The model under review builds one solid part; all positions refer to its coordinate system, in mm. Face numbers are marked on the shaded views. Round coordinates to 2 decimals unless told otherwise and drop trailing zeros. Order: outer loops, then holes, each group sorted by start corner. A loop starts at its lowest first (then second) coordinate and runs counter-clockwise, first axis right, second up.
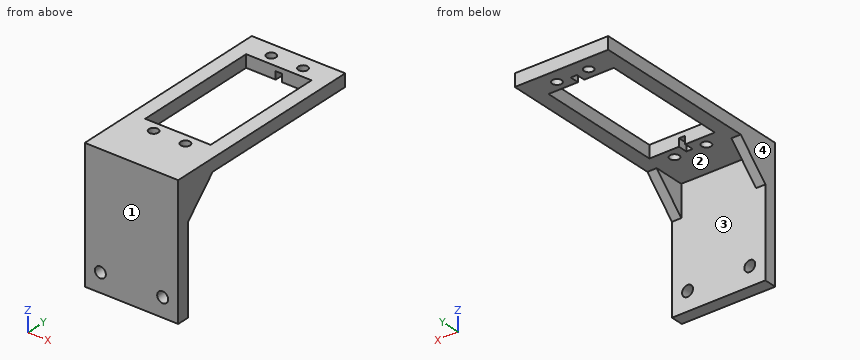
```python
from build123d import *

# Parameters (mm, degrees)
SKETCH_1_W          = 30
SKETCH_1_H          = 63.8558669
SKETCH_1_R          = 1.5
SKETCH_1_W_2        = 21
SKETCH_1_H_2        = 41
EXTRUDE_1_DEPTH     = 4
SKETCH_2_W          = 2
SKETCH_2_H          = 3
CUT_EXTRUDE_1_DEPTH = 2.5
SKETCH_3_W          = 30
SKETCH_3_H          = 42
EXTRUDE_2_DEPTH     = 4
SKETCH_4_R          = 1.75
CUT_EXTRUDE_2_DEPTH = 5
EXTRUDE_3_DEPTH     = 3
EXTRUDE_4_DEPTH     = 3


with BuildPart() as part:
    # 草圖1 → 填料-伸長1 (new body)
    with BuildSketch(Plane.XY):
        with Locations((15, 31.92793345)):
            Rectangle(SKETCH_1_W, SKETCH_1_H)
        with Locations((9.9, 59.2558669)):
            Circle(SKETCH_1_R, mode=Mode.SUBTRACT)
        with Locations((20.1, 59.2558669)):
            Circle(SKETCH_1_R, mode=Mode.SUBTRACT)
        with Locations((20.1, 11.4558669)):
            Circle(SKETCH_1_R, mode=Mode.SUBTRACT)
        with Locations((9.9, 11.4558669)):
            Circle(SKETCH_1_R, mode=Mode.SUBTRACT)
        with Locations((15, 35.3558669)):
            Rectangle(SKETCH_1_W_2, SKETCH_1_H_2, mode=Mode.SUBTRACT)
    extrude(amount=EXTRUDE_1_DEPTH)

    # 草圖2 → 除料-伸長1 (cut)
    with BuildSketch(Plane(origin=(0, 0, 0), x_dir=(-1, 0, 0), z_dir=(0, 0, -1))):
        with Locations((-15, 57.3558669)):
            Rectangle(SKETCH_2_W, SKETCH_2_H)
        with Locations((-15, 13.3558669)):
            Rectangle(SKETCH_2_W, SKETCH_2_H)
    extrude(amount=-CUT_EXTRUDE_1_DEPTH, mode=Mode.SUBTRACT)

    # 草圖3 → 填料-伸長2 (add)
    with BuildSketch(Plane.XZ):
        with Locations((15, -17)):
            Rectangle(SKETCH_3_W, SKETCH_3_H)
    extrude(amount=EXTRUDE_2_DEPTH)

    # 草圖4 → 除料-伸長2 (cut, through all)
    with BuildSketch(Plane(origin=(0, 0, 0), x_dir=(1, 0, 0), z_dir=(0, 1, 0))):
        with Locations((5, 32)):
            Circle(SKETCH_4_R)
        with Locations((25, 32)):
            Circle(SKETCH_4_R)
    extrude(amount=-CUT_EXTRUDE_2_DEPTH, mode=Mode.SUBTRACT)

    # 草圖5 → 填料-伸長3 (add)
    with BuildSketch(Plane(origin=(30, 0, 0), x_dir=(0, 0, -1), z_dir=(1, 0, 0))):
        Polygon((0, 10), (10, 0), (0, 0), align=None)
    extrude(amount=-EXTRUDE_3_DEPTH)

    # 草圖6 → 填料-伸長4 (add)
    with BuildSketch(Plane.ZY):
        Polygon((0, 0), (0, 10), (-10, 0), align=None)
    extrude(amount=-EXTRUDE_4_DEPTH)


solid = part.part
```
(1) Consider section B-B (x = 20.1). Write out the cut boundary in (y, z).
Data:
outline: (-4, -38) - (0, -38) - (0, 0) - (9.96, 0) - (9.96, 4) - (-4, 4) - close; (12.96, 0) - (14.86, 0) - (14.86, 4) - (12.96, 4) - close; (55.86, 0) - (57.76, 0) - (57.76, 4) - (55.86, 4) - close; (60.76, 0) - (63.86, 0) - (63.86, 4) - (60.76, 4) - close
(2) Consider section A-A (y = 52). Write out the cut boundary in (x, z), and give its area (3 significant figures).
Data:
outline: (0, 0) - (4.5, 0) - (4.5, 4) - (0, 4) - close; (25.5, 0) - (30, 0) - (30, 4) - (25.5, 4) - close
area: 36.0 mm2
(3) Consider section C-C (z = -32). Write out the cut boundary in (x, y), and give its area (3 significant figures).
Data:
outline: (0, -4) - (3.25, -4) - (3.25, 0) - (0, 0) - close; (6.75, -4) - (23.25, -4) - (23.25, 0) - (6.75, 0) - close; (26.75, -4) - (30, -4) - (30, 0) - (26.75, 0) - close
area: 92.0 mm2
(4) To check wall thickness, follow probe 1 along X at (y, z) = (-2.4, -32); probe 2 along Y at (x, z) = (9.9, 1.4); probe 3 along Z at (x, y) = (25, -2.95). State the ranges of each line that lie inside material, in increasing order.
Data:
probe 1: x = 0 to 3.25, 6.75 to 23.25, 26.75 to 30
probe 2: y = -4 to 9.96, 12.96 to 14.86, 55.86 to 57.76, 60.76 to 63.86
probe 3: z = -38 to -33.75, -30.25 to 4
(5) Consider section D-D (x = 5.25). Write out the cut boundary in (y, z), and give its area (3 significant figures).
Data:
outline: (-4, -38) - (0, -38) - (0, -33.73) - (-4, -33.73) - close; (-4, -30.27) - (0, -30.27) - (0, 0) - (14.86, 0) - (14.86, 4) - (-4, 4) - close; (55.86, 0) - (63.86, 0) - (63.86, 4) - (55.86, 4) - close
area: 246 mm2
(6) Draft analysis for pull direction X (two halves, no side actions). For the marked faces 1, 2, 3 and 4, state which applies: pulls with the +X half, pulls with the -X half, needs draft (parallel to the pull), parting line crosses it, or undercut.
Data:
face 1: needs draft
face 2: undercut
face 3: undercut
face 4: pulls with the -X half
(7) Insertion check: pin 1 (1.2 mm diameter, centred on y = 13, z = 1, fed in from -X); pin 2 (5 mm diameter, centred on x = 9.9, y = 11.46, fed in from -Z); pin 3 (0.6 mm diameter, centred on x = 14.5, y = 57, fed in from -Z); pin 4 (1 mm diameter, centred on x = 13, z = -12, fed in from +Y). Each pin has a flat end and moves straight along its axis. Give the tip position at first contact, or say it passes through.
Data:
pin 1: stops at x = 0
pin 2: stops at z = 0
pin 3: stops at z = 2.5
pin 4: stops at y = 0
